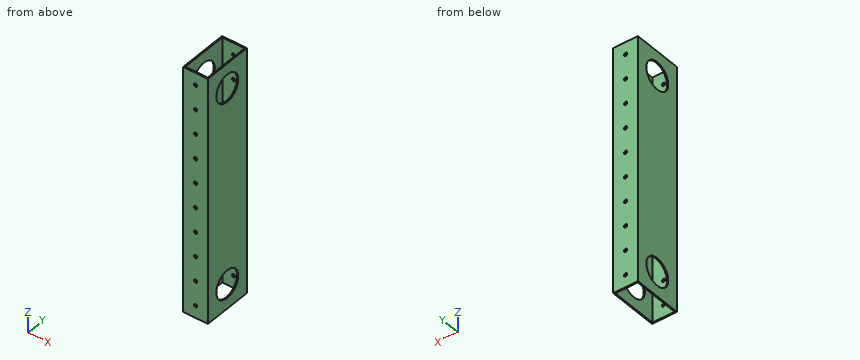
Autodesk Inventor part; units mm, degrees
ref_plane "YZ Plane" through (0, 0, 0) normal (1, 0, 0) x (0, 1, 0)
ref_plane "XZ Plane" through (0, 0, 0) normal (0, 1, 0) x (-1, 0, 0)
ref_plane "XY Plane" through (0, 0, 0) normal (0, 0, 1) x (1, 0, 0)
sketch "Sketch1" plane through (0, 0, 0) normal (0, 0, 1) x (1, 0, 0)
  line L0 (-12.1708, 16.0073) -> (13.2292, 16.0073)
  line L1 (13.2292, 16.0073) -> (13.2292, -34.7927)
  line L2 (13.2292, -34.7927) -> (-12.1708, -34.7927)
  line L3 (-12.1708, -34.7927) -> (-12.1708, 16.0073)
  line L4 (11.9592, 14.7373) -> (-10.9008, 14.7373)
  line L5 (-10.9008, 14.7373) -> (-10.9008, -33.5227)
  line L6 (-10.9008, -33.5227) -> (11.9592, -33.5227)
  line L7 (11.9592, -33.5227) -> (11.9592, 14.7373)
  point P0 (0, 0)
  dimension "d0" = 25.4
  dimension "d1" = 50.8
  dimension "d2" = 1.27
extrude "Extrusion1" add sketch "Sketch1" along normal blind 254
sketch "Sketch2" plane through (-12.1708, 16.0073, 0) normal (0, 1, 0) x (1, 0, 0)
  circle A0 centre (12.7, -12.7) radius 1.7272
  line L0 (25.4, 0) -> (0, 0)
  line L1 (0, 0) -> (0, -254)
  point P0 (12.1708, 0)
  dimension "d5" = 3.4544
  dimension "d6" = 12.7
  dimension "d7" = 12.7
extrude "Extrusion2" cut sketch "Sketch2" against normal through all
pattern_linear "Rectangular Pattern1" count 10 spacing 25.4 along (0, 0, 1) of "Extrusion2"
sketch "Sketch3" plane through (13.2292, -34.7927, 0) normal (1, 0, 0) x (0, 0, -1)
  circle A0 centre (-228.6, 25.4) radius 14.2875
  circle A1 centre (-25.4, 25.4) radius 14.2875
  line L0 (-228.6, 25.4) -> (-25.4, 25.4) construction
  line L1 (-254, 0) -> (-254, 50.8)
  line L2 (0, 0) -> (-254, 0)
  point P0 (0, 34.7927)
  dimension "d15" = 203.2
  dimension "d16" = 25.4
  dimension "d17" = 25.4
  dimension "d18" = 28.575
extrude "Extrusion3" cut sketch "Sketch3" against normal through all
equation "\"d3\" = d13"
equation "\"d13\" = 254"
properties part number "VerseFrame 10in KY"
Design review of the part built by this model. Coordinates are the model's own, in mm. Coordinates: 2 decimals unless noted, no trailing zeros. Order: outer loops, then holes, each group sorted by start corner. A loop starts at its lowest first (then second) coordinate and runs counter-clockwise, first axis right, second up. Notation, with made-up numbers: M 57.5,53.25 L 81.5,53.25 A29 cw 81.5,88.25 Z; hole C 88.25,-12 d8. An arc over 180 degrees is marked long. Answer as a JSON object with one key per item and string values. Group by question number.
1) Wall thickness on L1, parallel to Y at x = 8.25, z = 36.5; L2, parallel to Y at x = -11.5, z = 25.4; L3, parallel to X at y = -28, z = 61: over which ranges is each line inside the solid? List them lowest first.
2) Add section B-B, the plane x = 5. Write out the cut boundary in (y, z).
3) Add section A-A, the plane z = 25.4. Write out the cut boundary in (x, y), then the cut area to 3 significant figures.
4) For pin 1 (3 mm diameter, centred on x = 0.53, z = 12.7, fed in from -Y), flat-tipped, find the tip position at first contact; note if it passes through.
5) Add section D-D, the plane y = -20. Write out the cut boundary in (x, z).
6) Add section C-C, the plane z = 57. Write out the cut boundary in (x, y), then the cut area to 3 significant figures.
Computed values:
{
 "1": {"L1": "y = -34.79 to -33.52, 14.74 to 16.01", "L2": "y = -34.79 to -23.68, 4.89 to 16.01", "L3": "x = -12.17 to -10.9, 11.96 to 13.23"},
 "2": {"outline": "M -34.79,0 L -33.52,0 L -33.52,254 L -34.79,254 Z; M 14.74,0 L 16.01,0 L 16.01,254 L 14.74,254 Z"},
 "3": {"outline": "M -12.17,-34.79 L 13.23,-34.79 L 13.23,-23.68 L 11.96,-23.68 L 11.96,-33.52 L -10.9,-33.52 L -10.9,-23.68 L -12.17,-23.68 Z; M -12.17,4.89 L -10.9,4.89 L -10.9,14.74 L 11.96,14.74 L 11.96,4.89 L 13.23,4.89 L 13.23,16.01 L -12.17,16.01 Z", "area": "115 mm^2"},
 "4": {"pin 1": "passes through"},
 "5": {"outline": "M -12.17,0 L -10.9,0 L -10.9,15.83 L -12.17,15.83 Z; M -12.17,34.97 L -10.9,34.97 L -10.9,219.03 L -12.17,219.03 Z; M -12.17,238.17 L -10.9,238.17 L -10.9,254 L -12.17,254 Z; M 11.96,0 L 13.23,0 L 13.23,15.83 L 11.96,15.83 Z; M 11.96,34.97 L 13.23,34.97 L 13.23,219.03 L 11.96,219.03 Z; M 11.96,238.17 L 13.23,238.17 L 13.23,254 L 11.96,254 Z"},
 "6": {"outline": "M -12.17,-34.79 L 13.23,-34.79 L 13.23,16.01 L -12.17,16.01 Z; hole M -10.9,-33.52 L 11.96,-33.52 L 11.96,14.74 L -10.9,14.74 Z", "area": "187 mm^2"}
}
